```python
from build123d import *

# Parameters (mm, degrees)
CROQUIS1_W               = 90
CROQUIS1_H               = 120
SALIENTE_EXTRUIR1_DEPTH  = 15
VACIADO1_T               = -2
CROQUIS3_W               = 56.3
CROQUIS3_H               = 85.6
CORTAR_EXTRUIR1_DEPTH    = 10
CROQUIS4_R               = 2
SALIENTE_EXTRUIR2_DEPTH  = 3
CROQUIS5_R               = 1.5
SALIENTE_EXTRUIR3_DEPTH  = 2
CROQUIS6_R               = 5.5
CORTAR_EXTRUIR2_DEPTH    = 4
REDONDEO1_R              = 10
RANURA_START             = 43
RANURA_DE_RESORTE1_DEPTH = 2
CORTAR_EXTRUIR3_DEPTH    = 110.201648339


# Read off the part's stored shape, not the designer's step: Ranura de resorte1
with BuildPart() as part:
    # Croquis1 → Saliente-Extruir1 (new body)
    with BuildSketch(Plane(origin=(0, 0, 0), x_dir=(1, 0, 0), z_dir=(0, 1, 0))):
        Rectangle(CROQUIS1_W, CROQUIS1_H)
    extrude(amount=SALIENTE_EXTRUIR1_DEPTH)

    # Vaciado1
    vaciado1_openings = [part.faces().sort_by_distance(p)[0] for p in [
        (0, 0, 0),
    ]]
    offset(amount=VACIADO1_T, openings=vaciado1_openings, kind=Kind.INTERSECTION)

    # Croquis3 → Cortar-Extruir1 (cut)
    with BuildSketch(Plane(origin=(0, 15, 0), x_dir=(1, 0, 0), z_dir=(0, 1, 0))):
        with Locations((-0.189097346, 9.095595484)):
            Rectangle(CROQUIS3_W, CROQUIS3_H)
    extrude(amount=-CORTAR_EXTRUIR1_DEPTH, mode=Mode.SUBTRACT)

    # Croquis4 → Saliente-Extruir2 (add)
    with BuildSketch(Plane.XZ.offset(-13)):
        with Locations(Location((-23.989097346, 35.904404516, 0), (0, 0, 270))):
            Circle(CROQUIS4_R)
        with Locations(Location((23.610902654, 35.904404516, 0), (0, 0, 270))):
            Circle(CROQUIS4_R)
        with Locations(Location((-23.989097346, -54.095595484, 0), (0, 0, 270))):
            Circle(CROQUIS4_R)
        with Locations(Location((23.610902654, -54.095595484, 0), (0, 0, 270))):
            Circle(CROQUIS4_R)
    extrude(amount=SALIENTE_EXTRUIR2_DEPTH)

    # Croquis5 → Saliente-Extruir3 (add)
    with BuildSketch(Plane.XZ.offset(-10)):
        with Locations(Location((-23.989097346, -54.095595484, 0), (0, 0, 270))):
            Circle(CROQUIS5_R)
        with Locations(Location((23.610902654, -54.095595484, 0), (0, 0, 270))):
            Circle(CROQUIS5_R)
        with Locations(Location((23.610902654, 35.904404516, 0), (0, 0, 270))):
            Circle(CROQUIS5_R)
        with Locations(Location((-23.989097346, 35.904404516, 0), (0, 0, 270))):
            Circle(CROQUIS5_R)
    extrude(amount=SALIENTE_EXTRUIR3_DEPTH)

    # Croquis6 → Cortar-Extruir2 (cut)
    with BuildSketch(Plane(origin=(0, 15, 0), x_dir=(1, 0, 0), z_dir=(0, 1, 0))):
        with Locations(Location((-30, -47, 0), (0, 0, 270))):
            Circle(CROQUIS6_R)
        with Locations(Location((0, -47, 0), (0, 0, 270))):
            Circle(CROQUIS6_R)
        with Locations(Location((30, -47, 0), (0, 0, 270))):
            Circle(CROQUIS6_R)
    extrude(amount=-CORTAR_EXTRUIR2_DEPTH, mode=Mode.SUBTRACT)

    # Redondeo1
    redondeo1_edges = [part.edges().sort_by_distance(p)[0] for p in [
        (-43, 6.5, -58),
        (-43, 6.5, 58),
        (43, 6.5, 58),
        (43, 6.5, -58),
        (-45, 7.5, -60),
        (45, 7.5, -60),
        (45, 7.5, 60),
        (-45, 7.5, 60),
    ]]
    fillet(redondeo1_edges, radius=REDONDEO1_R)

    # Ranura de resorte1 outline → Ranura de resorte1 (cut)
    with BuildSketch(Plane.YZ.offset(RANURA_START)):
        Polygon((7, -38.234845775), (1, -37.9203991), (1, -42.549292451), (7, -42.234845775), align=None)
    extrude(amount=RANURA_DE_RESORTE1_DEPTH, mode=Mode.SUBTRACT)

    # Croquis7 → Cortar-Extruir3 (cut, through all)
    with BuildSketch(Plane(origin=(45, 0, 0), x_dir=(0, 0, -1), z_dir=(1, 0, 0))):
        Polygon((42.549292451, 1), (37.9203991, 1), (38.234845775, 7), (42.234845775, 7), align=None)
        Polygon((-42.234845775, 7), (-42.549292451, 1), (-37.9203991, 1), (-38.234845775, 7), align=None)
    extrude(amount=-CORTAR_EXTRUIR3_DEPTH, mode=Mode.SUBTRACT)


solid = part.part
```
Geometry: final body of the model. Coordinates: model frame, mm. A direction names the side the tool comes from. Round coordinates to 2 decimals unless told otherwise and drop trailing zeros. Write each loop counter-clockwise with the first axis right and the second up, starting at its lowest first coordinate (ties: lowest second). Pieces come first, ordered by that corner, then holes.
Item 1: Section query B-B (z = 8.5). Return loops of the section in (x, y), plus the area to 3 significant figures.
Item 2: Section query A-A (x = 30). Return loops of the section in (y, z), plus the area to 3 significant figures.
Item 3: Section query C-C (x = 0). Return loops of the section in (y, z).
Item 4: Set-up query: faces 1 (the face through (30.242, 14.014, 41.505)), 2 (the face through (40.15, 6.41, -54.99)). Return all of +Z, -Z, +X, -X, +Y, -Y with unobstructed straight access to the full face (end or side cutting, diameter ignored); none if empty.
Item 5: Section query D-D (y = 3.25). Give the number of separate pieces and of enclosed holes in the cut face, plus the area to 3 significant figures.
Item 6: Material intervals for L1, parallel to X at y = 13.8, z = 47; L2, parallel to Z at x = 30, y = 12; L3, parallel to X at y = 5.75, z = -2, sorted ascending.
Item 7: Mould query, pull axis Z, two halves, no side actions, for faces 3 (the face through (0, 7, -60)), 4 (the face through (41.99, 7.6, 57.15)), 5 (the face through (-25.21, 11.52, 37.49)). Classes: +Z half, -Z half, draft (parallel to the pull), parting line (faces both ways), or undercut.
Item 8: Pin query (flat end, axial travel): P1, Ø9, axis at x = -30, z = 47, coming from the +Y side; P2, Ø2.5, axis at x = 24, z = -54, coming from the -Y side. Return the tip coordinate at first contact, or that it passes through.
Completed:
1. outline: (-45, 0) - (-43, 0) - (-43, 13) - (-28.34, 13) - (-28.34, 15) - (-45, 15) - close; (27.96, 13) - (43, 13) - (43, 0) - (45, 0) - (45, 15) - (27.96, 15) - close
1. area: 119 mm2
2. outline: (0, -60) - (15, -60) - (15, 41.5) - (13, 41.5) - (13, -58) - (0, -58) - close; (0, 58) - (13, 58) - (13, 52.5) - (15, 52.5) - (15, 60) - (0, 60) - close
2. area: 270 mm2
3. outline: (0, -60) - (15, -60) - (15, -51.9) - (13, -51.9) - (13, -58) - (0, -58) - close; (0, 58) - (13, 58) - (13, 52.5) - (15, 52.5) - (15, 60) - (0, 60) - close; (13, 33.7) - (15, 33.7) - (15, 41.5) - (13, 41.5) - close
4. face 1: +Y, -Y
4. face 2: -Y
5. separate pieces: 4
5. enclosed holes: 0
5. area: 789 mm2
6. L1: x = -45 to -35.5, -24.5 to -5.5, 5.5 to 24.5, 35.5 to 45
6. L2: z = -60 to -58, 58 to 60
6. L3: x = -45 to -43, 43 to 45
7. face 3: -Z half
7. face 4: +Z half
7. face 5: undercut
8. P1: passes through
8. P2: stops at y = 8
